For this review, take the finished solid that the model builds, in its own axes (mm). A direction names the side the tool comes from. Coordinates: 2 decimals unless noted, no trailing zeros. Loops run counter-clockwise (first coordinate to the right, second up) from the corner with the lowest first, then second, coordinate; pieces in that order, holes last. Notation, with made-up numbers: (-28, 33) - (-11, 33) arc R35 ccw to (-11, 71) - close; hole circle Ø7 at (58, 48.5). An arc over 180 degrees is marked (long way). Answer as a JSON object with one key per item and string values. Group by question number.
Item 1: Mouldability with a two-part tool opening along Y and no side actions: class faces 4 (the flat face through (1, 23, 18)), 5 (the cylindrical face through (8.331, 12.526, 17.972)), 6 (the flat face through (20, 13, 18)), 7 (the cylindrical face through (10.228, 20.735, 17.972)) as released by +Y, released by -Y, zero draft, split by the parting line, or undercut.
Item 2: We need section A-A (z = 10). Give the boundary of the cut face in (x, y), then the cut area to 3 significant figures.
Item 3: Clearance check with flat-ended pins moving along their axes: pin 1 (4 mm diameter, centred on x = 10, y = 12, fed in from -Z); pin 2 (3 mm diameter, centred on x = 13, z = 4, fed in from +Y); pin 3 (3 mm diameter, centred on y = 11.5, z = 19, fed in from +X). State where each tip first meets the part, or that it passes through.
Item 4: We need section B-B (x = 10). Give the boundary of the cut face in (y, z), then the cut area to 3 significant figures.
Item 5: To check wall thickness, follow line 1 (X direction, y = 0.9, z = 10); line 2 (Y direction, x = 10, z = 18.2); line 3 (Y direction, x = 43.5, z = 3). State the ranges of each line that lie inside material, in increasing order.
Item 6: Tool access review of faces 1 (the cylindrical face through (56.669, 2.028, 9.474)), 2 (the flat face through (32, 4, 10)), 3 (the flat face through (10, 14, 16)): name each direction out of +Z, -Z, +X, -X, +Y, -Y from which nothing blocks a thin tool from reaching the whole face with its end or side.
Item 7: We need section D-D (y = 12). Give the boundary of the cut face in (x, z), then the cut area to 3 significant figures.
Item 8: We need section C-C (x = 55). Give the boundary of the cut face in (y, z).
from build123d import *

# Parameters (mm, degrees)
SCHIZZO1_W                   = 65
SCHIZZO1_H                   = 4
ESTRUSIONE_ESTRUSIONE1_DEPTH = 20
SCHIZZO2_W                   = 20
SCHIZZO2_H                   = 4
ESTRUSIONE_ESTRUSIONE2_DEPTH = 20
TAGLIO_ESTRUSIONE1_REACH     = 6
SCHIZZO6_R                   = 1.75
TAGLIO_ESTRUSIONE2_REACH     = 6
SCHIZZO7_R                   = 1.75
RACCORDO1_R                  = 1
RACCORDO2_R                  = 1
SMUSSO1_SIZE                 = 2
SMUSSO3_SIZE                 = 2


with BuildPart() as part:
    # Schizzo1 → Estrusione-Estrusione1 (new body)
    with BuildSketch(Plane.XY):
        with Locations((32.5, 2)):
            Rectangle(SCHIZZO1_W, SCHIZZO1_H)
    extrude(amount=ESTRUSIONE_ESTRUSIONE1_DEPTH)

    # Schizzo2 → Estrusione-Estrusione2 (add)
    with BuildSketch(Plane(origin=(0, 4, 0), x_dir=(1, 0, 0), z_dir=(0, 1, 0))):
        with Locations((10, -18)):
            Rectangle(SCHIZZO2_W, SCHIZZO2_H)
    extrude(amount=ESTRUSIONE_ESTRUSIONE2_DEPTH)

    # Schizzo6 → Taglio-Estrusione1 (cut, up to next)
    with BuildSketch(Plane(origin=(0, 4, 0), x_dir=(1, 0, 0), z_dir=(0, 1, 0)), mode=Mode.PRIVATE) as taglio_estrusione1_sk1:
        with Locations((15, -10)):
            Circle(SCHIZZO6_R)
    taglio_estrusione1_tool1 = extrude(taglio_estrusione1_sk1.sketch, amount=-TAGLIO_ESTRUSIONE1_REACH, mode=Mode.PRIVATE) & part.part
    add(taglio_estrusione1_tool1.solids().sort_by_distance((15, 4, 10))[0], mode=Mode.SUBTRACT)
    # Schizzo6 → Taglio-Estrusione1 (cut, up to next)
    with BuildSketch(Plane(origin=(0, 4, 0), x_dir=(1, 0, 0), z_dir=(0, 1, 0)), mode=Mode.PRIVATE) as taglio_estrusione1_sk2:
        with Locations((55, -10)):
            Circle(SCHIZZO6_R)
    taglio_estrusione1_tool2 = extrude(taglio_estrusione1_sk2.sketch, amount=-TAGLIO_ESTRUSIONE1_REACH, mode=Mode.PRIVATE) & part.part
    add(taglio_estrusione1_tool2.solids().sort_by_distance((55, 4, 10))[0], mode=Mode.SUBTRACT)

    # Schizzo7 → Taglio-Estrusione2 (cut, up to next)
    with BuildSketch(Plane(origin=(0, 0, 16), x_dir=(-1, 0, 0), z_dir=(0, 0, -1)), mode=Mode.PRIVATE) as taglio_estrusione2_sk1:
        with Locations((-10, 19)):
            Circle(SCHIZZO7_R)
    taglio_estrusione2_tool1 = extrude(taglio_estrusione2_sk1.sketch, amount=-TAGLIO_ESTRUSIONE2_REACH, mode=Mode.PRIVATE) & part.part
    add(taglio_estrusione2_tool1.solids().sort_by_distance((10, 19, 16))[0], mode=Mode.SUBTRACT)
    # Schizzo7 → Taglio-Estrusione2 (cut, up to next)
    with BuildSketch(Plane(origin=(0, 0, 16), x_dir=(-1, 0, 0), z_dir=(0, 0, -1)), mode=Mode.PRIVATE) as taglio_estrusione2_sk2:
        with Locations((-10, 12)):
            Circle(SCHIZZO7_R)
    taglio_estrusione2_tool2 = extrude(taglio_estrusione2_sk2.sketch, amount=-TAGLIO_ESTRUSIONE2_REACH, mode=Mode.PRIVATE) & part.part
    add(taglio_estrusione2_tool2.solids().sort_by_distance((10, 12, 16))[0], mode=Mode.SUBTRACT)

    # Raccordo1
    raccordo1_edges = [part.edges().sort_by_distance(p)[0] for p in [
        (10, 4, 16),
    ]]
    fillet(raccordo1_edges, radius=RACCORDO1_R)

    # Raccordo2
    raccordo2_edges = [part.edges().sort_by_distance(p)[0] for p in [
        (20, 4, 18),
    ]]
    fillet(raccordo2_edges, radius=RACCORDO2_R)

    # Smusso1
    smusso1_edges = [part.edges().sort_by_distance(p)[0] for p in [
        (0, 24, 18),
        (20, 24, 18),
    ]]
    chamfer(smusso1_edges, length=SMUSSO1_SIZE)

    # Smusso3
    smusso3_edges = [part.edges().sort_by_distance(p)[0] for p in [
        (0, 2, 0),
    ]]
    chamfer(smusso3_edges, length=SMUSSO3_SIZE)


solid = part.part
Check sheet entries:
{
 "1": {"face 4": "released by +Y", "face 5": "undercut", "face 6": "zero draft", "face 7": "undercut"},
 "2": {"outline": "(0, 0) - (13.25, 0) - (13.25, 4) - (0, 4) - close; (16.75, 0) - (53.25, 0) - (53.25, 4) - (16.75, 4) - close; (56.75, 0) - (65, 0) - (65, 4) - (56.75, 4) - close", "area": "232 mm2"},
 "3": {"pin 1": "stops at z = 16", "pin 2": "stops at y = 4", "pin 3": "stops at x = 20"},
 "4": {"outline": "(0, 0) - (4, 0) - (4, 15) arc R1 cw to (5, 16) - (10.25, 16) - (10.25, 20) - (0, 20) - close; (13.75, 16) - (17.25, 16) - (17.25, 20) - (13.75, 20) - close; (20.75, 16) - (24, 16) - (24, 20) - (20.75, 20) - close", "area": "132 mm2"},
 "5": {"line 1": "x = 0 to 13.25, 16.75 to 53.25, 56.75 to 65", "line 2": "y = 0 to 10.25, 13.75 to 17.25, 20.75 to 24", "line 3": "y = 0 to 4"},
 "6": {"face 1": "+Y, -Y", "face 2": "-Z, +X, +Y", "face 3": "-Z, +X, -X, +Y"},
 "7": {"outline": "(0, 16) - (8.25, 16) - (8.25, 20) - (0, 20) - close; (11.75, 16) - (20, 16) - (20, 20) - (11.75, 20) - close", "area": "66.0 mm2"},
 "8": {"outline": "(0, 0) - (4, 0) - (4, 8.25) - (0, 8.25) - close; (0, 11.75) - (4, 11.75) - (4, 20) - (0, 20) - close"}
}
